Answer from the drawing. Dimensions are ordinates in mm from the lowest x, y and z of the part. A direction names the side the tool comes from. Coordinates: 2 decimals unless noted, no trailing zeros. Order: outer loops, then holes, each group sorted by start corner. A loop starts at its lowest first (then second) coordinate and runs counter-clockwise, first axis right, second up. Notation, with made-up numbers: (23.5, 44.25) -> (68.5, 44.25) arc R17 cw to (68.5, 54.25) -> close; hole circle Ø10 at (78, -17.75). An arc over 180 degrees is marked (long way). Answer in a Markdown table with one row per item.
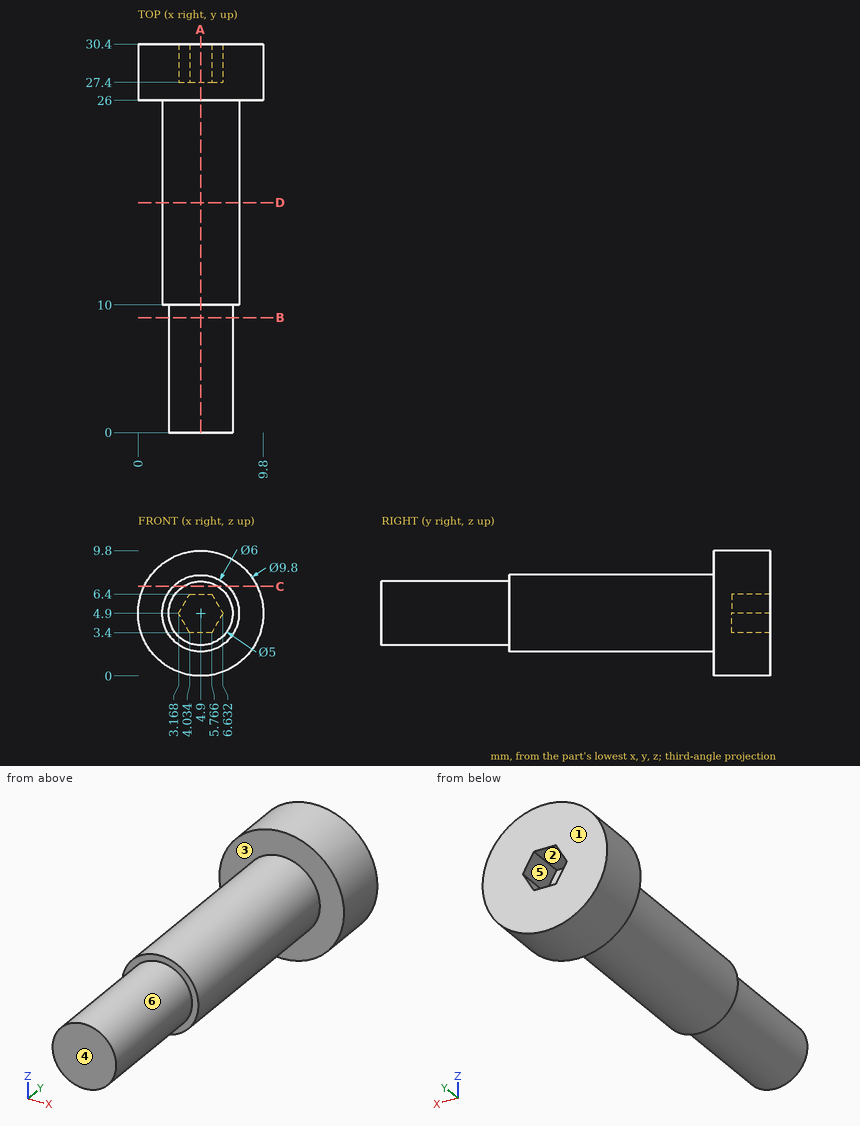
(1) Flat-ended cylindrical pins translate along their axes: pin 1 (5 mm diameter, centred on x = 5.5, z = 5.5, fed in from -Y); pin 2 (3 mm diameter, centred on x = 3.5, y = 22.5, fed in from -Z); pin 3 (4 mm diameter, centred on x = 5, y = 6.5, fed in from +Z); pin 4 (2 mm diameter, centred on y = 6, z = 8, fed in from +X). Find the tip coordinate at first contact, or state that the pin passes through.
Check values:
| item | result |
|---|---|
| pin 1 | y = 0 |
| pin 2 | z = 1.9 |
| pin 3 | z = 7.4 |
| pin 4 | x = 6.26 |
(2) A cutting plane is placed at C-C, the plane z = 7. Determine the outline of the cut face in (x, y).
Check values:
| item | result |
|---|---|
| outline | (0.47, 26) -> (2.76, 26) -> (2.76, 10) -> (3.54, 10) -> (3.54, 0) -> (6.26, 0) -> (6.26, 10) -> (7.04, 10) -> (7.04, 26) -> (9.33, 26) -> (9.33, 30.4) -> (0.47, 30.4) -> close |
(3) A cutting plane is placed at D-D, the plane y = 18. Determine the outline of the cut face in (x, z), then the cut area to 3 significant figures.
Check values:
| item | result |
|---|---|
| outline | circle Ø6 at (4.9, 4.9) |
| area | 28.3 mm² |
(4) Find the intervals of material crossed by line 1 along Y through (x, z) = (7.75, 8.5); line 2 along X through (y, z) = (2, 4.75); line 3 along Z through (x, y) = (7.5, 21.5), in increasing order. Write a range as from..to.
Check values:
| item | result |
|---|---|
| line 1 | 26..30.4 |
| line 2 | 2.4..7.4 |
| line 3 | 3.4..6.4 |
(5) For a pull along Z with two mould halves and no side action, classify the marked faces 4, 5 and 6 as released by +Z, released by -Z, zero draft, split by the parting line, or undercut.
Check values:
| item | result |
|---|---|
| face 4 | zero draft |
| face 5 | undercut |
| face 6 | split by the parting line |
(6) A cutting plane is placed at A-A, the plane x = 4.9. Determine the outline of the cut face in (y, z), then the cut area to 3 significant figures.
Check values:
| item | result |
|---|---|
| outline | (0, 2.4) -> (10, 2.4) -> (10, 1.9) -> (26, 1.9) -> (26, 0) -> (30.4, 0) -> (30.4, 3.4) -> (27.4, 3.4) -> (27.4, 6.4) -> (30.4, 6.4) -> (30.4, 9.8) -> (26, 9.8) -> (26, 7.9) -> (10, 7.9) -> (10, 7.4) -> (0, 7.4) -> close |
| area | 180 mm² |
(7) A cutting plane is placed at B-B, the plane y = 9. Determine the outline of the cut face in (x, z), then the cut area to 3 significant figures.
Check values:
| item | result |
|---|---|
| outline | circle Ø5 at (4.9, 4.9) |
| area | 19.6 mm² |
(8) Which of the six approach directions +Z, -Z, +X, -X, +Y, -Y give full straight-line access (tool end or side, diameter ignored) to the marked faces 1, 2 and 3?
Check values:
| item | result |
|---|---|
| face 1 | +Z, -Z, +X, -X, +Y |
| face 2 | +Y |
| face 3 | -Y |
